Read the model definition and answer for the solid it produces. Units are mm, in the model's axes. A direction names the side the tool comes from. Coordinates: 2 decimals unless noted, no trailing zeros. Loops run counter-clockwise (first coordinate to the right, second up) from the corner with the lowest first, then second, coordinate; pieces in that order, holes last.
from build123d import *

# Parameters (mm, degrees)
BOSS_EXTRUDE1_DEPTH = 20
SKETCH3_R           = 2.25
CUT_EXTRUDE1_DEPTH  = 33.015621187
SKETCH4_R           = 1.5
CUT_EXTRUDE2_DEPTH  = 33.015621187


with BuildPart() as part:
    # Sketch2 → Boss-Extrude1 (new body)
    with BuildSketch(Plane(origin=(0, 0, 0), x_dir=(1, 0, 0), z_dir=(0, 1, 0))):
        Polygon((-20, 0), (0, 0), (0, 15), (2, 15), (2, -2), (-20, -2), align=None)
    extrude(amount=BOSS_EXTRUDE1_DEPTH)

    # Sketch3 → Cut-Extrude1 (cut, through all)
    with BuildSketch(Plane(origin=(0, 0, 0), x_dir=(-1, 0, 0), z_dir=(0, 0, -1))):
        with Locations((13, 10)):
            Circle(SKETCH3_R)
    extrude(amount=-CUT_EXTRUDE1_DEPTH, mode=Mode.SUBTRACT)

    # Sketch4 → Cut-Extrude2 (cut, through all)
    with BuildSketch(Plane.ZY):
        with Locations((-5, 10)):
            Circle(SKETCH4_R)
    extrude(amount=-CUT_EXTRUDE2_DEPTH, mode=Mode.SUBTRACT)


solid = part.part
Q1. A cutting plane is placed at D-D (x = -10). Give the vertices of the cut face in (y, z), then the cut area to 3 significant figures.
Findings below:
outline: (0, 0) - (20, 0) - (20, 2) - (0, 2) - close
area: 40.0 mm2
Q2. A cutting plane is placed at C-C (z = -5). Give the vertices of the cut face in (x, y), then the cut area to 3 significant figures.
Findings below:
outline: (0, 0) - (2, 0) - (2, 8.5) - (0, 8.5) - close; (0, 11.5) - (2, 11.5) - (2, 20) - (0, 20) - close
area: 34.0 mm2
Q3. Flat-ended cylindrical pins translate along their axes: pin 1 Ø1.8 at (y, z) = (10, -5) entering from +X; pin 2 Ø8 at (x, y) = (-12, 4) entering from -Z. Find the tip coordinate at first contact, or state that the pin passes through.
Findings below:
pin 1: passes through
pin 2: stops at z = 0
Q4. A cutting plane is placed at A-A (y = 10). Give the vertices of the cut face in (x, z), then the cut area to 3 significant figures.
Findings below:
outline: (-20, 0) - (-15.25, 0) - (-15.25, 2) - (-20, 2) - close; (-10.75, 0) - (0, 0) - (0, -3.5) - (2, -3.5) - (2, 2) - (-10.75, 2) - close; (0, -15) - (2, -15) - (2, -6.5) - (0, -6.5) - close
area: 59.0 mm2
Q5. Which of the six approach directions +Z, -Z, +X, -X, +Y, -Y give full straight-line access (tool end or side, diameter ignored) to faces 1 (the face through (1, 10, -15)), 2 (the face through (0, 10, -7))?
Findings below:
face 1: -Z, +X, -X, +Y, -Y
face 2: -Z, -X, +Y, -Y
Q6. Determine the mould class of faces 3 (the face through (-9, 10, 2)), 4 (the face through (-4.1, 20, 0.4)), 5 (the face through (1, 9.1, -6.2)) for opening direction Z: +Z half, -Z half, draft (parallel to the pull), parting line (faces both ways), or undercut.
Findings below:
face 3: +Z half
face 4: draft
face 5: undercut
Q7. A cutting plane is placed at B-B (x = -13). Give the vertices of the cut face in (y, z).
Findings below:
outline: (0, 0) - (7.75, 0) - (7.75, 2) - (0, 2) - close; (12.25, 0) - (20, 0) - (20, 2) - (12.25, 2) - close
Q8. Straight lines are drawn through the part: probe 1 along Y at (x, z) = (-13, 0.4); probe 2 along Z at (x, y) = (-4.75, 6.5); probe 3 along Y at (x, z) = (0.7, -5). For each, find the intervals that lie inside material, in ascending order.
Findings below:
probe 1: y = 0 to 7.75, 12.25 to 20
probe 2: z = 0 to 2
probe 3: y = 0 to 8.5, 11.5 to 20
